from build123d import *

# Parameters (mm, degrees)
BOSS_EXTRUDE1_DEPTH = 6


with BuildPart() as part:
    # Sketch1 → Boss-Extrude1 (new body)
    with BuildSketch(Plane.XY):
        with BuildLine():
            Line((684.689802479, 51.1944), (668.919080645, 51.1944))
            ThreePointArc((668.919080645, 51.1944), (666.832798953, 50.738344179), (665.127101625, 49.453371481))
            Line((665.127101625, 49.453371481), (663.897823459, 48.023043832))
            ThreePointArc((663.897823459, 48.023043832), (663.001524805, 46.501902162), (662.689802479, 44.764072351))
            Line((662.689802479, 44.764072351), (662.689802479, 40.62305))
            Line((662.689802479, 40.62305), (656.339802479, 40.62305))
            Line((656.339802479, 40.62305), (656.339802479, 46.61745))
            Line((656.339802479, 46.61745), (643.639802479, 46.61745))
            Line((643.639802479, 46.61745), (643.639802479, 40.62305))
            Line((643.639802479, 40.62305), (637.289802479, 40.62305))
            Line((637.289802479, 40.62305), (637.289802479, 52.5444))
            ThreePointArc((637.289802479, 52.5444), (638.754268573, 56.079933906), (642.289802479, 57.5444))
            Line((642.289802479, 57.5444), (662.689802479, 57.5444))
            Line((662.689802479, 57.5444), (684.689802479, 57.5444))
            Line((684.689802479, 57.5444), (684.689802479, 51.1944))
        make_face()
    extrude(amount=BOSS_EXTRUDE1_DEPTH)


solid = part.part
Can you work these out from the model? Positions are in its coordinate system, mm. A direction names the side the tool comes from. Round coordinates to 2 decimals unless told otherwise and drop trailing zeros. Write each loop counter-clockwise with the first axis right and the second up, starting at its lowest first coordinate (ties: lowest second). Pieces come first, ordered by that corner, then holes. Notation, with made-up numbers: (76.25, 24) -> (96.25, 24) arc R12 ccw to (96.25, 30) -> close; hole circle Ø2 at (61, -38.75). An arc over 180 degrees is marked (long way). One line per question, with ' | ' between items. Start each with the question number.
1) Suppose I cut it at A-A on y = 43. Write out the boundary of the cut face in (x, z), then the cut area to 3 significant figures.
2) Suppose I cut it at D-D on y = 49. Write out the boundary of the cut face in (x, z).
3) I'm going to push flat-ended pins straight in: P1, Ø1.5, axis at x = 662, y = 44.5, coming from the -Z side; P2, Ø1.5, axis at x = 664, z = 4.5, coming from the -Y side; P3, Ø1, axis at x = 644.5, z = 2, coming from the -Y side; P4, Ø3, axis at x = 680, z = 3, coming from the -Y side. Where does each tip first touch, or does it pass through?
4) Suppose I cut it at C-C on x = 676. Write out the boundary of the cut face in (y, z).
5) On a 3-axis mill with a long thin cutter (end or side, diameter ignored), from which of +Z, -Z, +X, -X, +Y, -Y can I reach the whole of each face in a straight line? I mean faces 5 (the flat face through (677, 51.194, 3)), 6 (the flat face through (656.34, 44, 3)), 7 (the cylindrical face through (638.716, 56.041, 2.958)). Say none if no direction works.
6) If we mould it in two halves opening along X, with no side actions, what happens to faces 1 (the cylindrical face through (663, 46.5, 3)), 2 (the flat face through (643.64, 44, 3)), 3 (the flat face through (660, 40.623, 3)), 4 (the flat face through (650, 46.617, 3))? For each: released by +X, released by -X, zero draft, split by the parting line, or undercut.
7) I need wall thicknesses on line 1 (X direction, y = 44, z = 4.4); line 2 (Y direction, x = 647, z = 3.3); line 3 (X direction, y = 52.75, z = 2.85). Which ranges of each line are inside material? Lowest first, please. Write a range as [from, to].
8) Suppose I cut it at B-B on z = 3.3. Write out the boundary of the cut face in (x, y).
Return value:
1) outline: (637.29, 0) -> (643.64, 0) -> (643.64, 6) -> (637.29, 6) -> close; (656.34, 0) -> (662.69, 0) -> (662.69, 6) -> (656.34, 6) -> close | area: 76.2 mm2
2) outline: (637.29, 0) -> (664.74, 0) -> (664.74, 6) -> (637.29, 6) -> close
3) P1: stops at z = 0 | P2: stops at y = 47.06 | P3: stops at y = 46.62 | P4: stops at y = 51.19
4) outline: (51.19, 0) -> (57.54, 0) -> (57.54, 6) -> (51.19, 6) -> close
5) face 5: +Z, -Z, +X, -Y | face 6: +Z, -Z, -Y | face 7: +Z, -Z, -X, +Y
6) face 1: released by +X | face 2: undercut | face 3: zero draft | face 4: undercut
7) line 1: x = [637.29, 643.64], [656.34, 662.69] | line 2: y = [46.62, 57.54] | line 3: x = [637.29, 684.69]
8) outline: (637.29, 40.62) -> (643.64, 40.62) -> (643.64, 46.62) -> (656.34, 46.62) -> (656.34, 40.62) -> (662.69, 40.62) -> (662.69, 44.76) arc R5 cw to (663.9, 48.02) -> (665.13, 49.45) arc R5 cw to (668.92, 51.19) -> (684.69, 51.19) -> (684.69, 57.54) -> (642.29, 57.54) arc R5 ccw to (637.29, 52.54) -> close
